```python
from build123d import *

# Parameters (mm, degrees)
F0_W     = 168
F0_H     = 58.99848
F2_DEPTH = 15
F3_W     = 10
F3_H     = 10
F4_DEPTH = 25
F1_W     = 10
F1_H     = 10.166666
F5_DEPTH = 40


with BuildPart() as f2:
    # F0 (on Top) → F2 (new body)
    with BuildSketch(Plane.XY):
        Rectangle(F0_W, F0_H)
    extrude(amount=F2_DEPTH)

    # F3 (on Top) → F4 (join)
    with BuildSketch(Plane.XY):
        with Locations((-74, 0)):
            Rectangle(F3_W, F3_H)
        with Locations((-55.499591, 0)):
            Rectangle(F3_W, F3_H)
        with Locations((-36.999591, 0)):
            Rectangle(F3_W, F3_H)
        with Locations((-18.499591, 0)):
            Rectangle(F3_W, F3_H)
        with Locations((18.499591, 0)):
            Rectangle(F3_W, F3_H)
        with Locations((36.999591, 0)):
            Rectangle(F3_W, F3_H)
        with Locations((55.499591, 0)):
            Rectangle(F3_W, F3_H)
        with Locations((74, 0)):
            Rectangle(F3_W, F3_H)
    extrude(amount=F4_DEPTH)

    # F1 (on Top) → F5 (join)
    with BuildSketch(Plane.XY):
        Rectangle(F1_W, F1_H)
    extrude(amount=F5_DEPTH)


solid = f2.part
```
Model file for the job. Use its own axes, mm. A direction names the side the tool comes from. Coordinates: 2 decimals unless noted, no trailing zeros. Loops run counter-clockwise (first coordinate to the right, second up) from the corner with the lowest first, then second, coordinate; pieces in that order, holes last. Notation, with made-up numbers: (59.5, 24.5) - (111.5, 24.5) arc R10 cw to (111.5, 41.5) - close; hole circle Ø4 at (56, 77.5). An arc over 180 degrees is marked (long way). Answer as a JSON object with one key per item and string values. Group by question number.
(1) Tool access for faces 1 (the face through (-79, 0, 20)), 2 (the face through (32, 0, 20)): list every direction of +Z, -Z, +X, -X, +Y, -Y with a clear straight run to the whole face (end or side of a thin tool).
(2) Flat gauge pins, fed straight in: pin 1 (11 mm diameter, centred on x = 72.5, y = 2, fed in from +Z); pin 2 (1.5 mm diameter, centred on x = 47, y = 18, fed in from +Z); pin 3 (3 mm diameter, centred on x = 58, z = 20, fed in from -Y). Where does each tip first touch, or does it go through?
(3) Cut at A-A (x = 20.5). Give the cut face in (y, z), then the cut area to 3 significant figures.
(4) Cut at D-D (z = 30). Give the cut face in (x, y), then the cut area to 3 significant figures.
(5) Two-plate mould, pull along X, no slides. Class faces 3 (the face through (-69, 0, 20)), 4 (the face through (84, 0, 7)), 5 (the face through (55, 5, 20)): released by +X, released by -X, zero draft, split by the parting line, or undercut.
(6) Probe line 1 along Z through (x, y) = (74.5, -8); line 2 along X through (y, z) = (-4.5, 32.5). List the from-to ranges inside material, lowest first.
(7) Cut at B-B (z = 22.5). State how many separate pieces and enclosed holes the cut face has, then the cut area to 3 significant figures.
(8) Cut at C-C (y = 21). Give the cut face in (x, z), then the cut area to 3 significant figures.
Geometry says:
{
 "1": {"face 1": "+Z, -X, +Y, -Y", "face 2": "+Z, +Y, -Y"},
 "2": {"pin 1": "stops at z = 25", "pin 2": "stops at z = 15", "pin 3": "stops at y = -5"},
 "3": {"outline": "(-29.5, 0) - (29.5, 0) - (29.5, 15) - (5, 15) - (5, 25) - (-5, 25) - (-5, 15) - (-29.5, 15) - close", "area": "985 mm^2"},
 "4": {"outline": "(-5, -5.08) - (5, -5.08) - (5, 5.08) - (-5, 5.08) - close", "area": "102 mm^2"},
 "5": {"face 3": "undercut", "face 4": "released by +X", "face 5": "zero draft"},
 "6": {"line 1": "z = 0 to 15", "line 2": "x = -5 to 5"},
 "7": {"separate pieces": "9", "enclosed holes": "0", "area": "902 mm^2"},
 "8": {"outline": "(-84, 0) - (84, 0) - (84, 15) - (-84, 15) - close", "area": "2,520 mm^2"}
}
